For this review, take the finished solid that the model builds, in its own axes (mm). Give positions to 0.01 mm unless a question says otherwise; leave off trailing zeros. Write each loop counter-clockwise with the first axis right and the second up, starting at its lowest first coordinate (ties: lowest second). Pieces come first, ordered by that corner, then holes. Notation, with made-up numbers: M -9,-34 L 35,-34 A27 cw 35,-7 Z; hole C 51,79 d4. An arc over 180 degrees is marked long. One line per item, written item: value. Start each with the question number.
Item 1: To check wall thickness, follow probe 1 along X at (y, z) = (2, 1); probe 2 along Y at (x, z) = (-14, 11); probe 3 along X at (y, z) = (29, 12.5). State the ranges of each line that lie inside material, in increasing order.
Item 2: Clearance check with flat-ended pins moving along their axes: pin 1 Ø4 at (y, z) = (21.5, -6) entering from -X; pin 2 Ø1 at (y, z) = (29.5, 11.5) entering from -X; pin 3 Ø2 at (y, z) = (15, 10) entering from +X. State where each tip first meets the part, or that it passes through.
Item 3: Consider section A-A, the plane y = 3. Write out the cut boundary in (x, z).
```python
from build123d import *

# Parameters (mm, degrees)
BOSS_EXTRUDE1_DEPTH = 40
FILLET1_R           = 0.5


with BuildPart() as part:
    # Sketch1 → Boss-Extrude1 (new body)
    with BuildSketch(Plane(origin=(0, 0, 0), x_dir=(-1, 0, 0), z_dir=(0, 1, 0))):
        Polygon((-10.423602647, 18.05420848), (10.421696815, 18.05420848), (20.844346546, 0.001649597), (10.421696815, -18.050909286), (-10.423602647, -18.050909286), (-20.846252377, 0.001649597), align=None)
    extrude(amount=BOSS_EXTRUDE1_DEPTH)

    # Fillet1
    fillet1_edges = [part.edges().sort_by_distance(p)[0] for p in [
        (0.000952916, 40, -18.050909286),
        (-15.63302168, 40, -9.024629844),
        (-15.63302168, 40, 9.027929039),
        (0.000952916, 40, 18.05420848),
        (15.634927512, 40, 9.027929039),
        (0.000952916, 0, 18.05420848),
        (-15.63302168, 0, 9.027929039),
        (-15.63302168, 0, -9.024629844),
        (0.000952916, 0, -18.050909286),
        (15.634927512, 0, -9.024629844),
        (15.634927512, 0, 9.027929039),
        (15.634927512, 40, -9.024629844),
    ]]
    fillet(fillet1_edges, radius=FILLET1_R)


solid = part.part
```
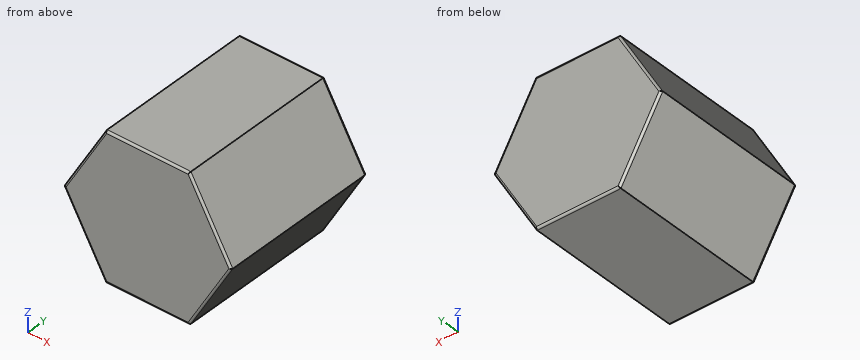
Model answer:
1. probe 1: x = -20.27 to 20.27
1. probe 2: y = 0.01 to 39.99
1. probe 3: x = -13.63 to 13.63
2. pin 1: stops at x = -18.53
2. pin 2: stops at x = -14.49
2. pin 3: stops at x = 15.65
3. outline: M -20.84,0 L -10.42,-18.05 L 10.42,-18.05 L 20.85,0 L 10.42,18.05 L -10.42,18.05 Z
